Check sheet for the modelled part. Datum: model origin and axes. Units: mm. A direction names the side the tool comes from. Coordinates: 2 decimals unless noted, no trailing zeros. Loops run counter-clockwise (first coordinate to the right, second up) from the corner with the lowest first, then second, coordinate; pieces in that order, holes last. Notation, with made-up numbers: (29.5, 38.25) - (36.5, 38.25) arc R13 cw to (36.5, 63.25) - close; hole circle Ø2 at (0, 79.5). An arc over 180 degrees is marked (long way). Answer as a JSON object with one key per item and string values. Group by question number.
from build123d import *

# Parameters (mm, degrees)
SKETCH1_W           = 195
SKETCH1_H           = 95
BOSS_EXTRUDE1_DEPTH = 1.6
SKETCH1_5_W         = 7.5
SKETCH1_5_H         = 2.5
SKETCH1_5_W_2       = 2.5
SKETCH1_5_W_3       = 10
BOSS_EXTRUDE2_DEPTH = 75
BOSS_EXTRUDE3_DEPTH = 20
CUT_EXTRUDE1_START  = 1.6
SKETCH1_7_W         = 2.5
SKETCH1_7_H         = 2.5
CUT_EXTRUDE1_DEPTH  = 5


with BuildPart() as part:
    # Sketch1 → Boss-Extrude1 (new body)
    with BuildSketch(Plane(origin=(0, 0, 0), x_dir=(1, 0, 0), z_dir=(0, 1, 0))):
        with Locations((100, 50)):
            Rectangle(SKETCH1_W, SKETCH1_H)
    extrude(amount=BOSS_EXTRUDE1_DEPTH)

    # Sketch1<5> → Boss-Extrude2 (add)
    with BuildSketch(Plane(origin=(0, 0, 0), x_dir=(1, 0, 0), z_dir=(0, 1, 0))):
        Polygon((0, 0), (100, 0), (100, 2.5), (2.5, 2.5), (2.5, 75), (2.5, 77.5), (0, 77.5), align=None)
        Polygon((100, 2.5), (100, 0), (200, 0), (200, 77.5), (197.5, 77.5), (197.5, 75), (197.5, 2.5), align=None)
        with Locations((193.75, 76.25)):
            Rectangle(SKETCH1_5_W, SKETCH1_5_H)
        with Locations((188.75, 76.25)):
            Rectangle(SKETCH1_5_W_2, SKETCH1_5_H)
        with Locations((182.5, 76.25)):
            Rectangle(SKETCH1_5_W_3, SKETCH1_5_H)
        with Locations((176.25, 76.25)):
            Rectangle(SKETCH1_5_W_2, SKETCH1_5_H)
        with Locations((170, 76.25)):
            Rectangle(SKETCH1_5_W_3, SKETCH1_5_H)
        with Locations((163.75, 76.25)):
            Rectangle(SKETCH1_5_W_2, SKETCH1_5_H)
        with Locations((157.5, 76.25)):
            Rectangle(SKETCH1_5_W_3, SKETCH1_5_H)
        with Locations((151.25, 76.25)):
            Rectangle(SKETCH1_5_W_2, SKETCH1_5_H)
        with Locations((145, 76.25)):
            Rectangle(SKETCH1_5_W_3, SKETCH1_5_H)
        with Locations((138.75, 76.25)):
            Rectangle(SKETCH1_5_W_2, SKETCH1_5_H)
        with Locations((132.5, 76.25)):
            Rectangle(SKETCH1_5_W_3, SKETCH1_5_H)
        with Locations((126.25, 76.25)):
            Rectangle(SKETCH1_5_W_2, SKETCH1_5_H)
        with Locations((120, 76.25)):
            Rectangle(SKETCH1_5_W_3, SKETCH1_5_H)
        with Locations((113.75, 76.25)):
            Rectangle(SKETCH1_5_W_2, SKETCH1_5_H)
        with Locations((107.5, 76.25)):
            Rectangle(SKETCH1_5_W_3, SKETCH1_5_H)
        with Locations((101.25, 76.25)):
            Rectangle(SKETCH1_5_W_2, SKETCH1_5_H)
        with Locations((95, 76.25)):
            Rectangle(SKETCH1_5_W_3, SKETCH1_5_H)
        with Locations((88.75, 76.25)):
            Rectangle(SKETCH1_5_W_2, SKETCH1_5_H)
        with Locations((82.5, 76.25)):
            Rectangle(SKETCH1_5_W_3, SKETCH1_5_H)
        with Locations((76.25, 76.25)):
            Rectangle(SKETCH1_5_W_2, SKETCH1_5_H)
        with Locations((70, 76.25)):
            Rectangle(SKETCH1_5_W_3, SKETCH1_5_H)
        with Locations((63.75, 76.25)):
            Rectangle(SKETCH1_5_W_2, SKETCH1_5_H)
        with Locations((57.5, 76.25)):
            Rectangle(SKETCH1_5_W_3, SKETCH1_5_H)
        with Locations((51.25, 76.25)):
            Rectangle(SKETCH1_5_W_2, SKETCH1_5_H)
        with Locations((45, 76.25)):
            Rectangle(SKETCH1_5_W_3, SKETCH1_5_H)
        with Locations((38.75, 76.25)):
            Rectangle(SKETCH1_5_W_2, SKETCH1_5_H)
        with Locations((32.5, 76.25)):
            Rectangle(SKETCH1_5_W_3, SKETCH1_5_H)
        with Locations((26.25, 76.25)):
            Rectangle(SKETCH1_5_W_2, SKETCH1_5_H)
        with Locations((20, 76.25)):
            Rectangle(SKETCH1_5_W_3, SKETCH1_5_H)
        with Locations((13.75, 76.25)):
            Rectangle(SKETCH1_5_W_2, SKETCH1_5_H)
        with Locations((7.5, 76.25)):
            Rectangle(SKETCH1_5_W_3, SKETCH1_5_H)
    extrude(amount=BOSS_EXTRUDE2_DEPTH)

    # Sketch1<6> → Boss-Extrude3 (add)
    with BuildSketch(Plane(origin=(0, 0, 0), x_dir=(1, 0, 0), z_dir=(0, 1, 0))):
        Polygon((0, 100), (0, 77.5), (2.5, 77.5), (2.5, 97.5), (197.5, 97.5), (197.5, 77.5), (200, 77.5), (200, 100), align=None)
    extrude(amount=BOSS_EXTRUDE3_DEPTH)

    # Sketch1<7> → Cut-Extrude1 (cut)
    with BuildSketch(Plane(origin=(0, 0, 0), x_dir=(1, 0, 0), z_dir=(0, 1, 0)).offset(CUT_EXTRUDE1_START)):
        with Locations((188.75, 76.25)):
            Rectangle(SKETCH1_7_W, SKETCH1_7_H)
        with Locations((176.25, 76.25)):
            Rectangle(SKETCH1_7_W, SKETCH1_7_H)
        with Locations((163.75, 76.25)):
            Rectangle(SKETCH1_7_W, SKETCH1_7_H)
        with Locations((151.25, 76.25)):
            Rectangle(SKETCH1_7_W, SKETCH1_7_H)
        with Locations((138.75, 76.25)):
            Rectangle(SKETCH1_7_W, SKETCH1_7_H)
        with Locations((126.25, 76.25)):
            Rectangle(SKETCH1_7_W, SKETCH1_7_H)
        with Locations((113.75, 76.25)):
            Rectangle(SKETCH1_7_W, SKETCH1_7_H)
        with Locations((101.25, 76.25)):
            Rectangle(SKETCH1_7_W, SKETCH1_7_H)
        with Locations((88.75, 76.25)):
            Rectangle(SKETCH1_7_W, SKETCH1_7_H)
        with Locations((76.25, 76.25)):
            Rectangle(SKETCH1_7_W, SKETCH1_7_H)
        with Locations((63.75, 76.25)):
            Rectangle(SKETCH1_7_W, SKETCH1_7_H)
        with Locations((51.25, 76.25)):
            Rectangle(SKETCH1_7_W, SKETCH1_7_H)
        with Locations((38.75, 76.25)):
            Rectangle(SKETCH1_7_W, SKETCH1_7_H)
        with Locations((26.25, 76.25)):
            Rectangle(SKETCH1_7_W, SKETCH1_7_H)
        with Locations((13.75, 76.25)):
            Rectangle(SKETCH1_7_W, SKETCH1_7_H)
    extrude(amount=CUT_EXTRUDE1_DEPTH, mode=Mode.SUBTRACT)


solid = part.part
1. Sectioned sample at A-A on y = 29. Record the cut outline in (x, z).
2. Sectioned sample at C-C on x = 93. Record the cut outline in (y, z).
3. Release check for a two-part mould opening along X. For faces 1 (the face through (99, 1.6, -51)), 2 (the face through (0, 37, -40)), 3 (the face through (99, 0, -51)) record: released by +X, released by -X, zero draft, split by the parting line, or undercut.
4. Access from +Z, -Z, +X, -X, +Y, -Y to the whole of each face (thin tool, end or side, straight path). Record for faces 4 (the face through (197.5, 38, -39)), 5 (the face through (100, 20, -99)), 6 (the face through (99, 37, 0)).
5. Material ranges on line 1 (Z direction, x = 149.5, y = 5); line 2 (X direction, y = 43, z = -25); line 3 (Z direction, x = 45, y = 53), recorded low to high.
6. Sectioned sample at D-D on z = -81. Record the cut outline in (x, y).
7. Gauge pin test, flat ends, axial feed: pin 1 (5 mm diameter, centred on x = 164, z = -28, fed in from -Y); pin 2 (1.5 mm diameter, centred on x = 125.5, z = -49, fed in from +Y). Record the tip position at first contact, or that the pin passes through.
8. Sectioned sample at B-B on y = 12.5. Record the cut outline in (x, z), plus the area to 3 significant figures.
Answers follow:
{
 "1": {"outline": "(0, -77.5) - (200, -77.5) - (200, 0) - (0, 0) - close; hole (2.5, -75) - (197.5, -75) - (197.5, -2.5) - (2.5, -2.5) - close"},
 "2": {"outline": "(0, -100) - (20, -100) - (20, -97.5) - (1.6, -97.5) - (1.6, -77.5) - (75, -77.5) - (75, -75) - (1.6, -75) - (1.6, -2.5) - (75, -2.5) - (75, 0) - (0, 0) - close"},
 "3": {"face 1": "undercut", "face 2": "released by -X", "face 3": "zero draft"},
 "4": {"face 4": "+Y", "face 5": "-Z, +X, -X, +Y", "face 6": "+Z, +X, -X, +Y, -Y"},
 "5": {"line 1": "z = -100 to -97.5, -77.5 to -75, -2.5 to 0", "line 2": "x = 0 to 2.5, 197.5 to 200", "line 3": "z = -77.5 to -75, -2.5 to 0"},
 "6": {"outline": "(0, 0) - (200, 0) - (200, 20) - (197.5, 20) - (197.5, 1.6) - (2.5, 1.6) - (2.5, 20) - (0, 20) - close"},
 "7": {"pin 1": "stops at y = 0", "pin 2": "stops at y = 1.6"},
 "8": {"outline": "(0, -100) - (200, -100) - (200, 0) - (0, 0) - close; hole (2.5, -97.5) - (197.5, -97.5) - (197.5, -77.5) - (2.5, -77.5) - close; hole (2.5, -75) - (197.5, -75) - (197.5, -2.5) - (2.5, -2.5) - close", "area": "1,960 mm^2"}
}
